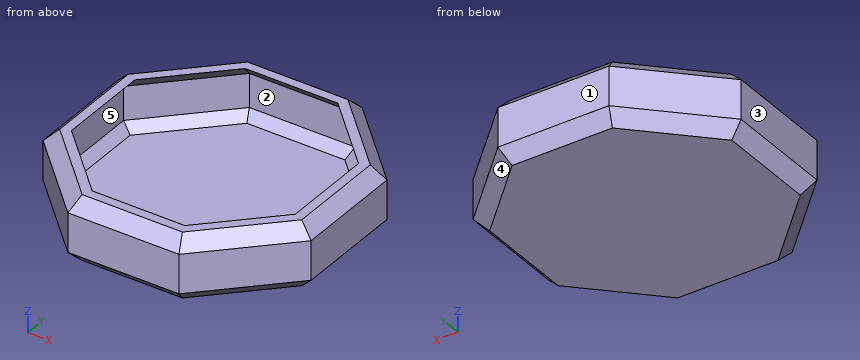
from build123d import *

# Parameters (mm, degrees)
F1_DEPTH = 25.4
F2_SIZE  = 5.08
F3_T     = -2.54


with BuildPart() as f1:
    # F0 (on Top) → F1 (new body)
    with BuildSketch(Plane.XY):
        Polygon((52.375846, -21.694786), (52.375846, 21.694786), (21.694786, 52.375846), (-21.694786, 52.375846), (-52.375846, 21.694786), (-52.375846, -21.694786), (-21.694786, -52.375846), (21.694786, -52.375846), align=None)
    extrude(amount=F1_DEPTH)

    # F2
    f2_edges = [f1.edges().sort_by_distance(p)[0] for p in [
        (37.035316, -37.035316, 25.4),
        (52.375846, 0, 25.4),
        (37.035316, 37.035316, 25.4),
        (0, 52.375846, 25.4),
        (-37.035316, 37.035316, 25.4),
        (-52.375846, 0, 25.4),
        (-37.035316, -37.035316, 25.4),
        (0, -52.375846, 25.4),
        (37.035316, -37.035316, 0),
        (52.375846, 0, 0),
        (37.035316, 37.035316, 0),
        (0, 52.375846, 0),
        (-37.035316, 37.035316, 0),
        (-52.375846, 0, 0),
        (-37.035316, -37.035316, 0),
        (0, -52.375846, 0),
    ]]
    chamfer(f2_edges, length=F2_SIZE)

    # F3
    f3_openings = [f1.faces().sort_by_distance(p)[0] for p in [
        (0, 0, 25.4),
    ]]
    offset(amount=F3_T, openings=f3_openings)


solid = f1.part
Input: part model. Units: mm. Frame: model coordinates. Face numbers are marked on the shaded views. A direction names the side the tool comes from. Give positions to 0.01 mm unless a question says otherwise; leave off trailing zeros. Write each loop counter-clockwise with the first axis right and the second up, starting at its lowest first coordinate (ties: lowest second). Pieces come first, ordered by that corner, then holes. Notation, with made-up numbers: M 0,30.5 L 17,30.5 A19 cw 17,60.5 Z; hole C 88.5,58 d9. An arc over 180 degrees is marked long. Write item = value, one per line. Start each with the question number.
1) Reachability of the marked faces 4 and 5 from +Z, -Z, +X, -X, +Y, -Y: full face, straight path, thin tool, end or side. Return the list, or none.
2) Cut plane B-B on z = 12.75. Return the cut outline in (x, y).
3) First-contact query: pin 1 Ø2 at (x, y) = (-35.5, 8.5) entering from +Z; pin 2 Ø3 at (y, z) = (-25.5, 21.5) entering from -X; pin 3 Ø6 at (x, z) = (35.5, 8.5) entering from -Y. Flat tips, straight axial feed; report the tip coordinate or a pass-through.
4) Draft query along X for the marked faces 1, 2 and 3. Return one class per face: +X half, -X half, draft (parallel to the pull), parting line (faces both ways), or undercut.
5) Material intervals for line 1 along Y through (x, z) = (-19, 12.25); line 2 along Z through (x, y) = (-9, 42.5), sorted ascending. Write a range as [from, to].
6) Cut plane A-A on x = -4. Return the cut outline in (y, z), then the cut area to 3 significant figures.
Solved:
q1.face_4 = -Z, +X, +Y
q1.face_5 = none
q2.outline = M -52.38,-21.69 L -21.69,-52.38 L 21.69,-52.38 L 52.38,-21.69 L 52.38,21.69 L 21.69,52.38 L -21.69,52.38 L -52.38,21.69 Z; hole M -49.84,-20.64 L -20.64,-49.84 L 20.64,-49.84 L 49.84,-20.64 L 49.84,20.64 L 20.64,49.84 L -20.64,49.84 L -49.84,20.64 Z
q3.pin_1 = 2.54
q3.pin_2 = -49.5
q3.pin_3 = -41.57
q4.face_1 = draft
q4.face_2 = undercut
q4.face_3 = -X half
q5.line_1 = [-52.38, -49.84], [49.84, 52.38]
q5.line_2 = [0, 2.54]
q6.outline = M -52.38,5.08 L -47.3,0 L 47.3,0 L 52.38,5.08 L 52.38,20.32 L 47.3,25.4 L 43.7,25.4 L 49.84,19.27 L 49.84,6.13 L 46.24,2.54 L -46.24,2.54 L -49.84,6.13 L -49.84,19.27 L -43.7,25.4 L -47.3,25.4 L -52.38,20.32 Z
q6.area = 381 mm2
